Drawing for the job (mm, zero at the part's lowest x, y, z). A direction names the side the tool comes from. Round coordinates to 2 decimals unless told otherwise and drop trailing zeros. Loops run counter-clockwise (first coordinate to the right, second up) from the corner with the lowest first, then second, coordinate; pieces in that order, holes last. Notation, with made-up numbers: M 32,5 L 36,5 A14 ccw 36,22 Z; hole C 82.5,63 d4. An arc over 180 degrees is marked long. Use a Markdown table: item, result. Add a question column.
Q1. Tool access for the marked faces 1 and 2: list every direction of +Z, -Z, +X, -X, +Y, -Y with a clear straight run to the whole face (end or side of a thin tool).
Q2. Cut at C-C (y = 70). Give the cut face in (x, z) (1 decimal).
Q3. Cut at A-A (z = 1). Give the cut face in (x, y).
Q4. Probe line 1 (Y direction, x = 39.5, z = 8); line 2 (Z direction, x = 30, y = 48.5). List the from-to ranges inside material, lowest first. Write a range as from..to.
Q5. Pin check, flat tip, straight feed: pin 1 (4 mm diameter, centred on x = 53, y = 48, fed in from -Z). Stop position of the tip, or through.
Q6. Cut at B-B (x = 27.5). Give the cut face in (y, z) (1 decimal).
Q7. Cut at D-D (x = 13). Give the cut face in (y, z).
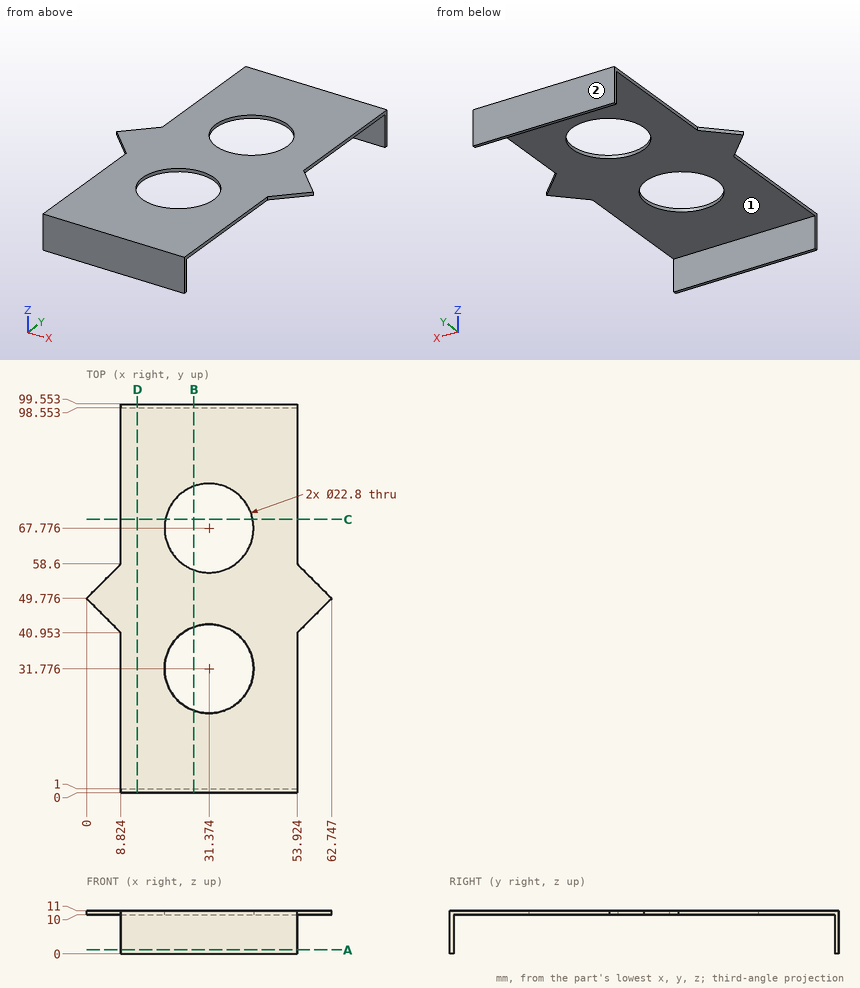
Checked values:
| question | item | result |
|---|---|---|
| 1 | face 1 | -Z, +X, -X |
| 1 | face 2 | +Z, -Z, +X, -X, +Y |
| 2 | outline | M 8.8,10 L 20.2,10 L 20.2,11 L 8.8,11 Z; M 42.6,10 L 53.9,10 L 53.9,11 L 42.6,11 Z |
| 3 | outline | M 8.82,0 L 53.92,0 L 53.92,1 L 8.82,1 Z; M 8.82,98.55 L 53.92,98.55 L 53.92,99.55 L 8.82,99.55 Z |
| 4 | line 1 | y = 0..1, 98.55..99.55 |
| 4 | line 2 | z = 10..11 |
| 5 | pin 1 | stops at z = 10 |
| 6 | outline | M 0,0 L 1,0 L 1,10 L 21.1,10 L 21.1,11 L 0,11 Z; M 42.5,10 L 57.1,10 L 57.1,11 L 42.5,11 Z; M 78.5,10 L 98.6,10 L 98.6,0 L 99.6,0 L 99.6,11 L 78.5,11 Z |
| 7 | outline | M 0,0 L 1,0 L 1,10 L 98.55,10 L 98.55,0 L 99.55,0 L 99.55,11 L 0,11 Z |
